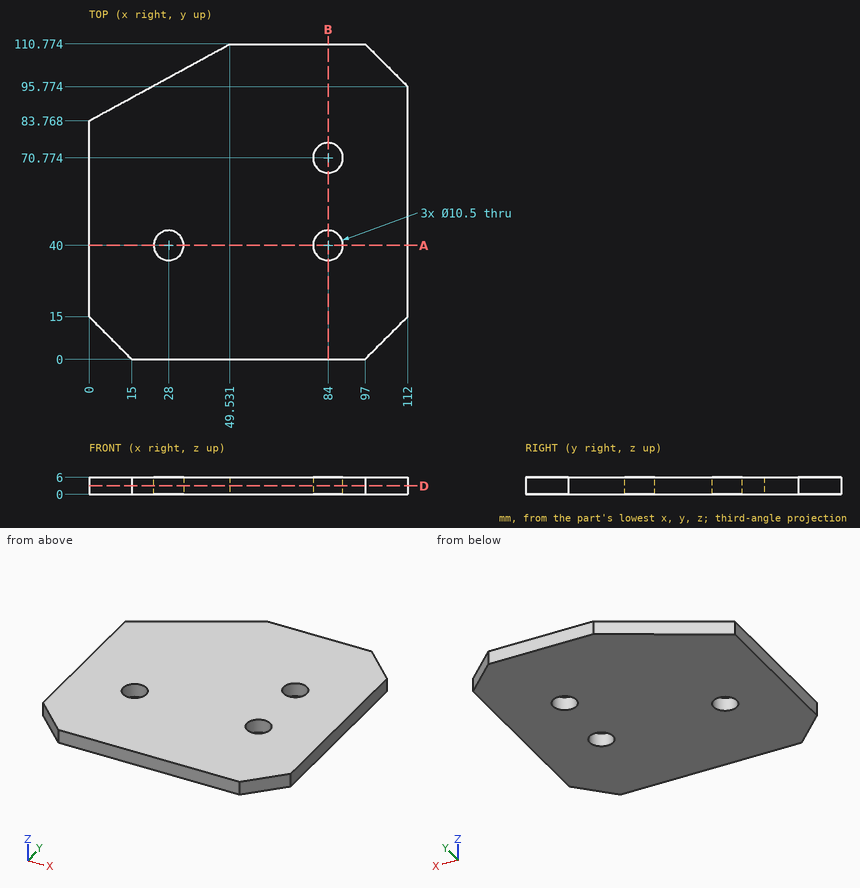
For this review, use the dimensioned drawing (mm, ordinates from the lowest corner) and the shaded views. Coordinates: 2 decimals unless noted, no trailing zeros. Loops run counter-clockwise (first coordinate to the right, second up) from the corner with the lowest first, then second, coordinate; pieces in that order, holes last. Notation, with made-up numbers: (38, -2.5) -> (90, -2.5) arc R23 ccw to (90, 35.5) -> close; hole circle Ø10 at (44.25, -35.75). An arc over 180 degrees is marked (long way). Use a Markdown table: item, result. Add a question column.
Item 1: We need section B-B, the plane x = 84. Write out the cut boundary in (y, z).
Item 2: We need section A-A, the plane y = 40. Write out the cut boundary in (x, z).
Item 3: We need section D-D, the plane z = 2.95. Write out the cut boundary in (x, y), and give its area (3 significant figures).
Item 4: Wall thickness on L1, parallel to Y at x = 84, z = 4.7; L2, parallel to X at y = 39, z = 2.2 (1 decimal); L3, parallel to Y at x = 81, z = 4.2 (1 decimal): over which ranges is each line inside the solid? List them lowest first. Write a range as from..to.
Item 5: Clearance check with a flat-ended pin moving along its axis: P1, Ø13.5, axis at x = 84, y = 70.77, coming from the -Z side. State where the tip first meets the part, or that it passes through.
Numbers:
| question | item | result |
|---|---|---|
| 1 | outline | (0, 0) -> (34.75, 0) -> (34.75, 6) -> (0, 6) -> close; (45.25, 0) -> (65.52, 0) -> (65.52, 6) -> (45.25, 6) -> close; (76.02, 0) -> (110.77, 0) -> (110.77, 6) -> (76.02, 6) -> close |
| 2 | outline | (0, 0) -> (22.75, 0) -> (22.75, 6) -> (0, 6) -> close; (33.25, 0) -> (78.75, 0) -> (78.75, 6) -> (33.25, 6) -> close; (89.25, 0) -> (112, 0) -> (112, 6) -> (89.25, 6) -> close |
| 3 | outline | (0, 15) -> (15, 0) -> (97, 0) -> (112, 15) -> (112, 95.77) -> (97, 110.77) -> (49.53, 110.77) -> (0, 83.77) -> close; hole circle Ø10.5 at (28, 40); hole circle Ø10.5 at (84, 40); hole circle Ø10.5 at (84, 70.77) |
| 3 | area | 11,100 mm^2 |
| 4 | L1 | y = 0..34.75, 45.25..65.52, 76.02..110.77 |
| 4 | L2 | x = 0..22.8, 33.2..78.8, 89.2..112 |
| 4 | L3 | y = 0..35.7, 44.3..66.5, 75.1..110.8 |
| 5 | P1 | stops at z = 0 |
